Part model, mm, in its own coordinate system. A direction names the side the tool comes from. Round coordinates to 2 decimals unless told otherwise and drop trailing zeros. Write each question's results on one line, items separated by ' | '. Start each with the question number.
(1) Tool access for faces 4 (the face through (21, 110, 0)), 5 (the face through (-21, 110, 0)), 6 (the face through (20, 7, 0)): list every direction of +Z, -Z, +X, -X, +Y, -Y with a clear straight run to the whole face (end or side of a thin tool).
(2) Flat gauge pins, fed straight in: P1, Ø4, axis at x = 22.5, z = -1.5, coming from the +Y side; P2, Ø8, axis at x = -6.5, z = 0, coming from the -Y side; P3, Ø10.5, axis at x = 17, y = 65, coming from the -Z side; P4, Ø1.2, axis at y = -2, z = -13, coming from the -X side. Where does each tip first touch, or does it go through?
(3) Drill centre lines: L1, parallel to X at y = 42.5, z = 0; L2, parallel to Y at x = -15.5, z = -13; L3, parallel to X at y = 64, z = -14. Where is each one in solid material? Low to high.
(4) Mould opens along Z. For faces 1 (the face through (22, 59, 15)), 2 (the face through (0, 100, 0)), 3 (the face through (24, 10, 0)) say: released by +Z, released by -Z, zero draft, split by the parting line, or undercut.
from build123d import *

# Parameters (mm, degrees)
FILLET_ON_TOP_EDGE_R                 = 3
SKETCH7_R                            = 7
CUT_FOR_WIRES_DEPTH                  = 150.507360339
SKETCH8_R                            = 19.424285286
CUT_FOR_HOLLOW_INSIDE_DEPTH          = 105
SKETCH9_R                            = 8
CUT_FOR_SIDE_BUTTON_DEPTH            = 150.507360339
RIGHT_PCB_PLATE_REACH                = 158.103
SKETCH10_W                           = 30
SKETCH10_H                           = 100
CUTS_FOR_BODY_SCREW_HOLES_DEPTH      = 150.548404931
CUTS_FOR_BODY_SCREW_HOLES_DEPTH_BACK = 150.548404931
SKETCH11_R                           = 1


with BuildPart() as part:
    # Sketch2 → Main Body (revolve)
    with BuildSketch(Plane.XY):
        with BuildLine():
            Line((0, 145), (0, -5))
            Line((0, -5), (21.424285286, -5))
            add(Edge.make_bspline(
                [(10.712142643, 145), (33.843636783, 71.251754866), (21.424285286, -5)],
                knots=[0, 0, 0, 1, 1, 1], degree=2))
            Line((10.712142643, 145), (0, 145))
        make_face()
    revolve(axis=Axis((0, 145, 0), (0, -1, 0)))

    # Fillet on Top Edge
    fillet_on_top_edge_edges = [part.edges().sort_by_distance(p)[0] for p in [
        (-10.712142643, 145, 0),
    ]]
    fillet(fillet_on_top_edge_edges, radius=FILLET_ON_TOP_EDGE_R)

    # Sketch7 → Cut for Wires (cut, through all)
    with BuildSketch(Plane(origin=(0, 0, 0), x_dir=(0, 0, -1), z_dir=(1, 0, 0))):
        Circle(SKETCH7_R)
    extrude(amount=CUT_FOR_WIRES_DEPTH, mode=Mode.SUBTRACT)

    # Sketch8 → Cut for Hollow Inside (cut)
    with BuildSketch(Plane.XZ.offset(5)):
        with Locations(Location((0, 0, 0), (0, 0, 270))):
            Circle(SKETCH8_R)
    extrude(amount=-CUT_FOR_HOLLOW_INSIDE_DEPTH, mode=Mode.SUBTRACT)

    # Sketch9 → Cut for Side Button (cut, through all)
    with BuildSketch(Plane.XY):
        with Locations(Location((0, 60, 0), (0, 0, 180))):
            Circle(SKETCH9_R)
    extrude(amount=CUT_FOR_SIDE_BUTTON_DEPTH, mode=Mode.SUBTRACT)

    # Sketch10 → Right PCB Plate (add, up to next)
    with BuildSketch(Plane(origin=(-26, 0, 0), x_dir=(0, 0, -1), z_dir=(1, 0, 0)), mode=Mode.PRIVATE) as right_pcb_plate_sk1:
        with Locations((0, 60)):
            Rectangle(SKETCH10_W, SKETCH10_H)
    right_pcb_plate_tool1 = extrude(right_pcb_plate_sk1.sketch, amount=RIGHT_PCB_PLATE_REACH, mode=Mode.PRIVATE) - part.part
    right_pcb_plate = right_pcb_plate_tool1.solids().sort_by_distance((-26, 60, 0))[0]
    add(right_pcb_plate)

    # Left PCB Plate: Right PCB Plate across plane
    add(right_pcb_plate.mirror(Plane(origin=(0, 0, 0), x_dir=(0, 0, 1), z_dir=(1, 0, 0))))

    # Sketch11 → Cuts for Body Screw Holes (cut, two sides: drawn at the far end of the back side and taken through both)
    with BuildSketch(Plane(origin=(0, 0, 0), x_dir=(0, 0, -1), z_dir=(1, 0, 0)).offset(-CUTS_FOR_BODY_SCREW_HOLES_DEPTH_BACK)):
        with Locations((-13, -2)):
            Circle(SKETCH11_R)
        with Locations((13, -2)):
            Circle(SKETCH11_R)
    extrude(amount=CUTS_FOR_BODY_SCREW_HOLES_DEPTH + CUTS_FOR_BODY_SCREW_HOLES_DEPTH_BACK, mode=Mode.SUBTRACT)


solid = part.part
A:
1) face 4: +X, +Y | face 5: -X, +Y | face 6: +X
2) P1: y = 110 | P2: y = 100 | P3: z = -22.43 | P4: through
3) L1: -26 to -19.42, 19.42 to 26 | L2: -5 to -3, -1 to 110 | L3: -26 to -13.46, 13.46 to 26
4) face 1: released by +Z | face 2: undercut | face 3: zero draft
